Verification items for this drawing (mm, ordinates from the low corner). A direction names the side the tool comes from. Give positions to 0.01 mm unless a question says otherwise; leave off trailing zeros. Write each loop counter-clockwise with the first axis right and the second up, starting at its lowest first coordinate (ties: lowest second). Pieces come first, ordered by that corner, then holes. Notation, with made-up numbers: (80, 33.25) -> (91, 33.25) arc R15 cw to (91, 50.25) -> close; hole circle Ø8 at (88, 41.5). An arc over 180 degrees is marked (long way). Use one line per item in the form item = value. Start each with the question number.
(1) Depth check by flat-ended pin: pin 1 Ø3 at (x, y) = (48, 3.5) entering from +Z; pin 2 Ø1 at (y, z) = (8.5, 30) entering from +X; pin 3 Ø7 at (x, z) = (30, 12.5) entering from -Y. Enter the tip coordinate at first touch or a pass-through.
(2) Section check A-A, the plane x = 30. Record the cut outline in (y, z).
(3) Scan lines: L1, parallel to Y at x = 36, z = 28.5; L2, parallel to Y at x = 24, z = 31 (1 decimal); L3, parallel to X at y = 1.5, z = 12.5. Record each from-to range of solid material in increasing order.
(4) Set-up check for the marked faces 1, 2, 3 and 4: record each of +Z, -Z, +X, -X, +Y, -Y from which the full face is reachable in a straight line by a thin tool's end or side.
(5) Section check D-D, the plane x = 43.5. Record the cut outline in (y, z), plus the area to 3 significant figures.
(6) Section check C-C, the plane z = 12.5. Record the cut outline in (x, y), plus the area to 3 significant figures.
(7) Section check B-B, the plane y = 1.5. Record the cut outline in (x, z), plus the area to 3 significant figures.
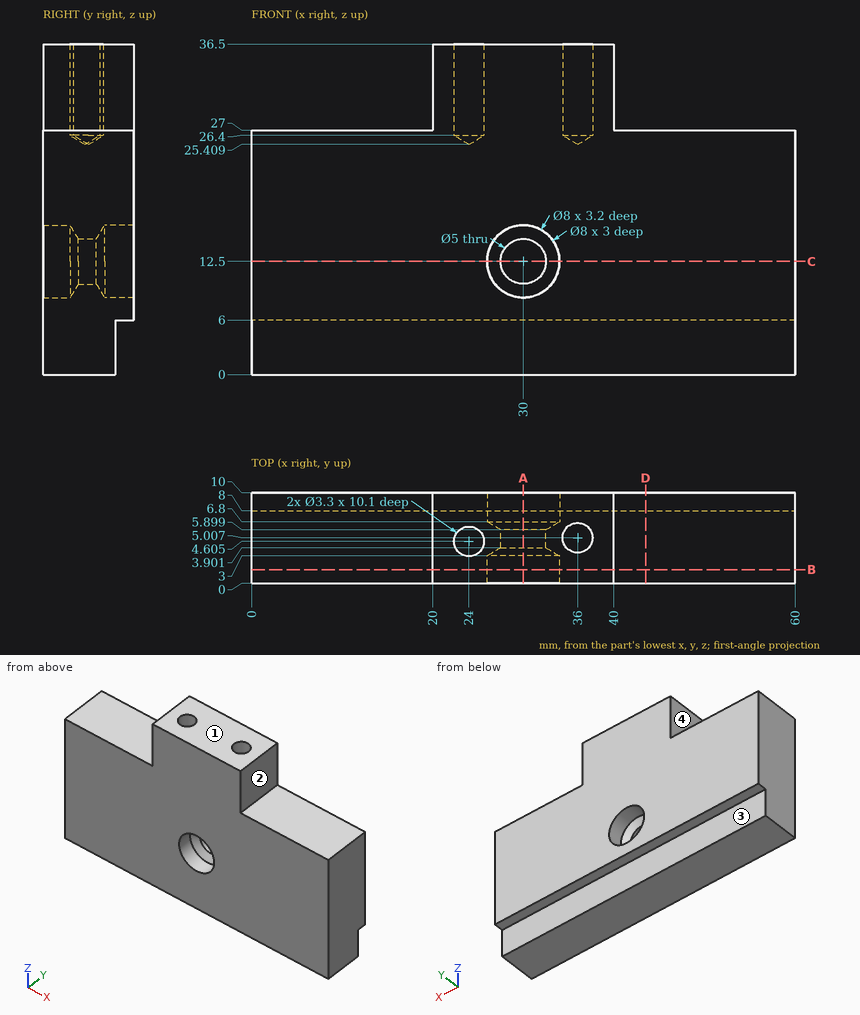
Completed:
q1.pin_1 = 27
q1.pin_2 = 40
q1.pin_3 = 3.3
q2.outline = (0, 0) -> (8, 0) -> (8, 6) -> (10, 6) -> (10, 8.5) -> (6.8, 8.5) -> (5.9, 10) -> (3.9, 10) -> (3, 8.5) -> (0, 8.5) -> close; (0, 16.5) -> (3, 16.5) -> (3.9, 15) -> (5.9, 15) -> (6.8, 16.5) -> (10, 16.5) -> (10, 36.5) -> (0, 36.5) -> close
q3.L1 = 0 to 3.36, 6.66 to 10
q3.L2 = 0 to 3, 6.3 to 10
q3.L3 = 0 to 26, 34 to 60
q4.face_1 = +Z, +X, -X, +Y, -Y
q4.face_2 = +Z, +X, +Y, -Y
q4.face_3 = -Z, +X, -X, +Y
q4.face_4 = +Z, -X, +Y, -Y
q5.outline = (0, 0) -> (8, 0) -> (8, 6) -> (10, 6) -> (10, 27) -> (0, 27) -> close
q5.area = 258 mm²
q6.outline = (0, 0) -> (26, 0) -> (26, 3) -> (27.5, 3.9) -> (27.5, 5.9) -> (26, 6.8) -> (26, 10) -> (0, 10) -> close; (32.5, 3.9) -> (34, 3) -> (34, 0) -> (60, 0) -> (60, 10) -> (34, 10) -> (34, 6.8) -> (32.5, 5.9) -> close
q6.area = 529 mm²
q7.outline = (0, 0) -> (60, 0) -> (60, 27) -> (40, 27) -> (40, 36.5) -> (20, 36.5) -> (20, 27) -> (0, 27) -> close; hole circle Ø8 at (30, 12.5)
q7.area = 1,760 mm²
